Source: CAD feature listing. Evaluate the final solid. Frame: model axes, mm. Round coordinates to 2 decimals unless told otherwise and drop trailing zeros. Write each loop counter-clockwise with the first axis right and the second up, starting at its lowest first coordinate (ties: lowest second). Pieces come first, ordered by that corner, then holes. Notation, with made-up numbers: M 4.25,46.25 L 57.25,46.25 A19 ccw 57.25,50.25 Z; hole C -6.75,6 d4. An arc over 180 degrees is marked long. Use a Markdown table: item, result.
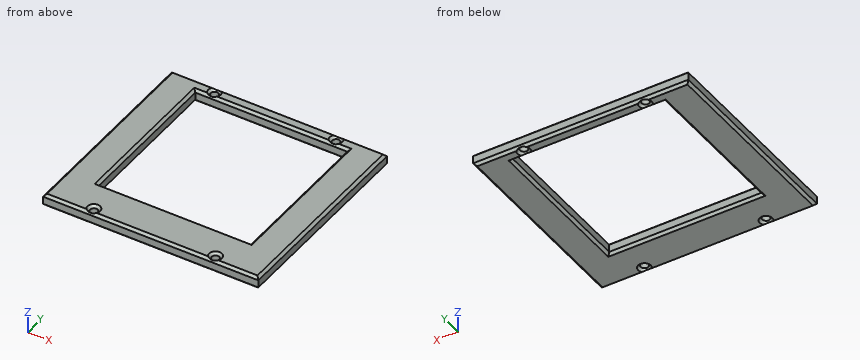
```python
from build123d import *

# Parameters (mm, degrees)
F0_W          = 85
F0_H          = 80
F0_R          = 1.5
F0_W_2        = 60
F0_H_2        = 60
F1_DEPTH      = 5
F2_T1_DEPTH   = 90.1433659759
F2_T3_DEPTH   = 85.1433659759
F2_T5_DEPTH   = 60
F2_T7_DEPTH   = 60
F2_T29_DEPTH  = 62.571682988
F2_T33_DEPTH  = 62.571682988
F2_T40_DEPTH  = 62.571682988
F2_T44_DEPTH  = 62.571682988
F2_T51_DEPTH  = 62.571682988
F2_T55_DEPTH  = 62.571682988
F2_T62_DEPTH  = 62.571682988
F2_T66_DEPTH  = 62.571682988
F2_T73_DEPTH  = 62.571682988
F2_T77_DEPTH  = 62.571682988
F2_T84_DEPTH  = 62.571682988
F2_T88_DEPTH  = 62.571682988
F2_T95_DEPTH  = 62.571682988
F2_T99_DEPTH  = 62.571682988
F2_T106_DEPTH = 62.571682988
F2_T110_DEPTH = 62.571682988


# Not quite as in the source:
# - a fillet or chamfer that OpenCascade refuses, or shapes differently, is made with other operations: its cross-section is extruded or revolved along the edge and cut away or added


with BuildPart() as f1:
    # F0 (on Top) → F1 (new body)
    with BuildSketch(Plane.XY):
        Rectangle(F0_W, F0_H)
        with Locations((-24, -37.5)):
            Circle(F0_R, mode=Mode.SUBTRACT)
        with Locations((24, -37.5)):
            Circle(F0_R, mode=Mode.SUBTRACT)
        with Locations((-24, 37.5)):
            Circle(F0_R, mode=Mode.SUBTRACT)
        with Locations((0, 5)):
            Rectangle(F0_W_2, F0_H_2, mode=Mode.SUBTRACT)
        with Locations((24, 37.5)):
            Circle(F0_R, mode=Mode.SUBTRACT)
    extrude(amount=F1_DEPTH)

    # F2: chamfer of 1 on 24 edges, made by hand

    # F2_s2 → F2_t1 (cut)
    with BuildSketch(Plane.YZ.offset(-45.071682988)):
        Polygon((40, 4), (39, 5), (40, 5), align=None)
        Polygon((-40, 4), (-39, 5), (-40, 5), align=None)
        Polygon((40, 1), (39, 0), (40, 0), align=None)
        Polygon((-40, 1), (-39, 0), (-40, 0), align=None)
    extrude(amount=F2_T1_DEPTH, mode=Mode.SUBTRACT)

    # F2_s4 → F2_t3 (cut)
    with BuildSketch(Plane.XZ.offset(-42.571682988)):
        Polygon((-42.5, 4), (-41.5, 5), (-42.5, 5), align=None)
        Polygon((42.5, 4), (41.5, 5), (42.5, 5), align=None)
        Polygon((-42.5, 1), (-41.5, 0), (-42.5, 0), align=None)
        Polygon((42.5, 1), (41.5, 0), (42.5, 0), align=None)
    extrude(amount=F2_T3_DEPTH, mode=Mode.SUBTRACT)

    # F2_s6 → F2_t5 (cut)
    with BuildSketch(Plane.XZ.offset(-35)):
        Polygon((-30, 4), (-31, 5), (-30, 5), align=None)
        Polygon((30, 4), (31, 5), (30, 5), align=None)
        Polygon((-30, 1), (-31, 0), (-30, 0), align=None)
        Polygon((30, 1), (31, 0), (30, 0), align=None)
    extrude(amount=F2_T5_DEPTH, mode=Mode.SUBTRACT)

    # F2_s8 → F2_t7 (cut)
    with BuildSketch(Plane.YZ.offset(-30)):
        Polygon((35, 4), (36, 5), (35, 5), align=None)
        Polygon((-25, 4), (-26, 5), (-25, 5), align=None)
        Polygon((35, 1), (36, 0), (35, 0), align=None)
        Polygon((-25, 1), (-26, 0), (-25, 0), align=None)
    extrude(amount=F2_T7_DEPTH, mode=Mode.SUBTRACT)

    # F2_s9 → F2_t10 (revolve, cut)
    with BuildSketch(Plane.XZ.offset(37.5)):
        Polygon((-22.5, 4), (-21.5, 5), (-22.5, 5), align=None)
    revolve(axis=Axis((-24, -37.5, 5), (0, 0, 1)), mode=Mode.SUBTRACT)

    # F2_s11 → F2_t12 (revolve, cut)
    with BuildSketch(Plane.XZ.offset(37.5)):
        Polygon((25.5, 4), (26.5, 5), (25.5, 5), align=None)
    revolve(axis=Axis((24, -37.5, 5), (0, 0, 1)), mode=Mode.SUBTRACT)

    # F2_s13 → F2_t14 (revolve, cut)
    with BuildSketch(Plane.XZ.offset(-37.5)):
        Polygon((-22.5, 4), (-21.5, 5), (-22.5, 5), align=None)
    revolve(axis=Axis((-24, 37.5, 5), (0, 0, 1)), mode=Mode.SUBTRACT)

    # F2_s15 → F2_t16 (revolve, cut)
    with BuildSketch(Plane.XZ.offset(-37.5)):
        Polygon((25.5, 4), (26.5, 5), (25.5, 5), align=None)
    revolve(axis=Axis((24, 37.5, 5), (0, 0, 1)), mode=Mode.SUBTRACT)

    # F2_s17 → F2_t18 (revolve, cut)
    with BuildSketch(Plane.XZ.offset(37.5)):
        Polygon((-22.5, 1), (-21.5, 0), (-22.5, 0), align=None)
    revolve(axis=Axis((-24, -37.5, 0), (0, 0, 1)), mode=Mode.SUBTRACT)

    # F2_s19 → F2_t20 (revolve, cut)
    with BuildSketch(Plane.XZ.offset(37.5)):
        Polygon((25.5, 1), (26.5, 0), (25.5, 0), align=None)
    revolve(axis=Axis((24, -37.5, 0), (0, 0, 1)), mode=Mode.SUBTRACT)

    # F2_s21 → F2_t22 (revolve, cut)
    with BuildSketch(Plane.XZ.offset(-37.5)):
        Polygon((-22.5, 1), (-21.5, 0), (-22.5, 0), align=None)
    revolve(axis=Axis((-24, 37.5, 0), (0, 0, 1)), mode=Mode.SUBTRACT)

    # F2_s23 → F2_t24 (revolve, cut)
    with BuildSketch(Plane.XZ.offset(-37.5)):
        Polygon((25.5, 1), (26.5, 0), (25.5, 0), align=None)
    revolve(axis=Axis((24, 37.5, 0), (0, 0, 1)), mode=Mode.SUBTRACT)


with BuildPart() as f2_tool27:
    # F2_s28 → F2_t29 (new body)
    with BuildSketch(Plane.XZ.offset(27.571682988)):
        Polygon((-30, 4), (-31, 5), (-30, 5), align=None)
    extrude(amount=-F2_T29_DEPTH)

    split(bisect_by=Plane.XZ.offset(25), keep=Keep.TOP)


with BuildPart() as f2_tool31:
    # F2_s32 → F2_t33 (new body)
    with BuildSketch(Plane.YZ.offset(30)):
        Polygon((-25, 4), (-26, 5), (-25, 5), align=None)
    extrude(amount=-F2_T33_DEPTH)

    split(bisect_by=Plane.YZ.offset(-30), keep=Keep.BOTTOM)


with BuildPart() as f2_tool27_1:
    add(f2_tool27.part)

    # F2_t35: intersect F2_tool31
    add(f2_tool31.part, mode=Mode.INTERSECT)


with BuildPart() as f1_1:
    add(f1.part)

    # F2_t25: cut F2_tool27
    add(f2_tool27_1.part, mode=Mode.SUBTRACT)


with BuildPart() as f2_tool38:
    # F2_s39 → F2_t40 (new body)
    with BuildSketch(Plane.XZ.offset(25)):
        Polygon((-30, 4), (-31, 5), (-30, 5), align=None)
    extrude(amount=-F2_T40_DEPTH)

    split(bisect_by=Plane.XZ.offset(-35), keep=Keep.BOTTOM)


with BuildPart() as f2_tool42:
    # F2_s43 → F2_t44 (new body)
    with BuildSketch(Plane.YZ.offset(-32.571682988)):
        Polygon((35, 4), (36, 5), (35, 5), align=None)
    extrude(amount=F2_T44_DEPTH)

    split(bisect_by=Plane.YZ.offset(-30), keep=Keep.BOTTOM)


with BuildPart() as f2_tool38_1:
    add(f2_tool38.part)

    # F2_t46: intersect F2_tool42
    add(f2_tool42.part, mode=Mode.INTERSECT)


with BuildPart() as f1_2:
    add(f1_1.part)

    # F2_t36: cut F2_tool38
    add(f2_tool38_1.part, mode=Mode.SUBTRACT)


with BuildPart() as f2_tool49:
    # F2_s50 → F2_t51 (new body)
    with BuildSketch(Plane.YZ.offset(-30)):
        Polygon((35, 4), (36, 5), (35, 5), align=None)
    extrude(amount=F2_T51_DEPTH)

    split(bisect_by=Plane.YZ.offset(30), keep=Keep.TOP)


with BuildPart() as f2_tool53:
    # F2_s54 → F2_t55 (new body)
    with BuildSketch(Plane.XZ.offset(-37.571682988)):
        Polygon((30, 4), (31, 5), (30, 5), align=None)
    extrude(amount=F2_T55_DEPTH)

    split(bisect_by=Plane.XZ.offset(-35), keep=Keep.BOTTOM)


with BuildPart() as f2_tool49_1:
    add(f2_tool49.part)

    # F2_t57: intersect F2_tool53
    add(f2_tool53.part, mode=Mode.INTERSECT)


with BuildPart() as f1_3:
    add(f1_2.part)

    # F2_t47: cut F2_tool49
    add(f2_tool49_1.part, mode=Mode.SUBTRACT)


with BuildPart() as f2_tool60:
    # F2_s61 → F2_t62 (new body)
    with BuildSketch(Plane.XZ.offset(-35)):
        Polygon((30, 4), (31, 5), (30, 5), align=None)
    extrude(amount=F2_T62_DEPTH)

    split(bisect_by=Plane.XZ.offset(25), keep=Keep.TOP)


with BuildPart() as f2_tool64:
    # F2_s65 → F2_t66 (new body)
    with BuildSketch(Plane.YZ.offset(32.571682988)):
        Polygon((-25, 4), (-26, 5), (-25, 5), align=None)
    extrude(amount=-F2_T66_DEPTH)

    split(bisect_by=Plane.YZ.offset(30), keep=Keep.TOP)


with BuildPart() as f2_tool60_1:
    add(f2_tool60.part)

    # F2_t68: intersect F2_tool64
    add(f2_tool64.part, mode=Mode.INTERSECT)


with BuildPart() as f1_4:
    add(f1_3.part)

    # F2_t58: cut F2_tool60
    add(f2_tool60_1.part, mode=Mode.SUBTRACT)


with BuildPart() as f2_tool71:
    # F2_s72 → F2_t73 (new body)
    with BuildSketch(Plane.XZ.offset(27.571682988)):
        Polygon((-30, 1), (-31, 0), (-30, 0), align=None)
    extrude(amount=-F2_T73_DEPTH)

    split(bisect_by=Plane.XZ.offset(25), keep=Keep.TOP)


with BuildPart() as f2_tool75:
    # F2_s76 → F2_t77 (new body)
    with BuildSketch(Plane.YZ.offset(30)):
        Polygon((-25, 1), (-26, 0), (-25, 0), align=None)
    extrude(amount=-F2_T77_DEPTH)

    split(bisect_by=Plane.YZ.offset(-30), keep=Keep.BOTTOM)


with BuildPart() as f2_tool71_1:
    add(f2_tool71.part)

    # F2_t79: intersect F2_tool75
    add(f2_tool75.part, mode=Mode.INTERSECT)


with BuildPart() as f1_5:
    add(f1_4.part)

    # F2_t69: cut F2_tool71
    add(f2_tool71_1.part, mode=Mode.SUBTRACT)


with BuildPart() as f2_tool82:
    # F2_s83 → F2_t84 (new body)
    with BuildSketch(Plane.XZ.offset(25)):
        Polygon((-30, 1), (-31, 0), (-30, 0), align=None)
    extrude(amount=-F2_T84_DEPTH)

    split(bisect_by=Plane.XZ.offset(-35), keep=Keep.BOTTOM)


with BuildPart() as f2_tool86:
    # F2_s87 → F2_t88 (new body)
    with BuildSketch(Plane.YZ.offset(-32.571682988)):
        Polygon((35, 1), (36, 0), (35, 0), align=None)
    extrude(amount=F2_T88_DEPTH)

    split(bisect_by=Plane.YZ.offset(-30), keep=Keep.BOTTOM)


with BuildPart() as f2_tool82_1:
    add(f2_tool82.part)

    # F2_t90: intersect F2_tool86
    add(f2_tool86.part, mode=Mode.INTERSECT)


with BuildPart() as f1_6:
    add(f1_5.part)

    # F2_t80: cut F2_tool82
    add(f2_tool82_1.part, mode=Mode.SUBTRACT)


with BuildPart() as f2_tool93:
    # F2_s94 → F2_t95 (new body)
    with BuildSketch(Plane.YZ.offset(-30)):
        Polygon((35, 1), (36, 0), (35, 0), align=None)
    extrude(amount=F2_T95_DEPTH)

    split(bisect_by=Plane.YZ.offset(30), keep=Keep.TOP)


with BuildPart() as f2_tool97:
    # F2_s98 → F2_t99 (new body)
    with BuildSketch(Plane.XZ.offset(-37.571682988)):
        Polygon((30, 1), (31, 0), (30, 0), align=None)
    extrude(amount=F2_T99_DEPTH)

    split(bisect_by=Plane.XZ.offset(-35), keep=Keep.BOTTOM)


with BuildPart() as f2_tool93_1:
    add(f2_tool93.part)

    # F2_t101: intersect F2_tool97
    add(f2_tool97.part, mode=Mode.INTERSECT)


with BuildPart() as f1_7:
    add(f1_6.part)

    # F2_t91: cut F2_tool93
    add(f2_tool93_1.part, mode=Mode.SUBTRACT)


with BuildPart() as f2_tool104:
    # F2_s105 → F2_t106 (new body)
    with BuildSketch(Plane.XZ.offset(-35)):
        Polygon((30, 1), (31, 0), (30, 0), align=None)
    extrude(amount=F2_T106_DEPTH)

    split(bisect_by=Plane.XZ.offset(25), keep=Keep.TOP)


with BuildPart() as f2_tool108:
    # F2_s109 → F2_t110 (new body)
    with BuildSketch(Plane.YZ.offset(32.571682988)):
        Polygon((-25, 1), (-26, 0), (-25, 0), align=None)
    extrude(amount=-F2_T110_DEPTH)

    split(bisect_by=Plane.YZ.offset(30), keep=Keep.TOP)


with BuildPart() as f2_tool104_1:
    add(f2_tool104.part)

    # F2_t112: intersect F2_tool108
    add(f2_tool108.part, mode=Mode.INTERSECT)


with BuildPart() as f1_8:
    add(f1_7.part)

    # F2_t102: cut F2_tool104
    add(f2_tool104_1.part, mode=Mode.SUBTRACT)


solid = f1_8.part
```
Q1. Section A-A on y = 30.5. Return loops of the section in (x, z).
Results are:
| item | result |
|---|---|
| outline | M -42.5,1 L -41.5,0 L -31,0 L -30,1 L -30,4 L -31,5 L -41.5,5 L -42.5,4 Z; M 30,1 L 31,0 L 41.5,0 L 42.5,1 L 42.5,4 L 41.5,5 L 31,5 L 30,4 Z |
Q2. First-contact query: pin 1 Ø1.8 at (x, y) = (-24, 37.5) entering from -Z; pin 2 Ø3.5 at (x, y) = (-24, -37.5) entering from +Z. Flat tips, straight axial feed; report the tip coordinate or a pass-through.
Results are:
| item | result |
|---|---|
| pin 1 | through |
| pin 2 | z = 4.25 |
Q3. Section B-B on x = -29. Return loops of the section in (y, z).
Results are:
| item | result |
|---|---|
| outline | M -40,1 L -39,0 L -26,0 L -25,1 L -25,4 L -26,5 L -39,5 L -40,4 Z; M 35,1 L 36,0 L 39,0 L 40,1 L 40,4 L 39,5 L 36,5 L 35,4 Z |
Q4. Line query: L1, parallel to Y at x = -24, z = 2.8; L2, parallel to Y at x = 3.5, z = 2.4; L3, parallel to X at y = 13.5, z = 1.4. Output: solid intervals per line, ascending.
Results are:
| item | result |
|---|---|
| L1 | -40 to -39, -36 to -25, 35 to 36, 39 to 40 |
| L2 | -40 to -25, 35 to 40 |
| L3 | -42.5 to -30, 30 to 42.5 |
